Could you check a few things on this model? Use its own coordinates, in mm. A direction names the side the tool comes from. Round coordinates to 2 decimals unless told otherwise and drop trailing zeros. Loops run counter-clockwise (first coordinate to the right, second up) from the corner with the lowest first, then second, coordinate; pieces in that order, holes last. Notation, with made-up numbers: (39.25, 52.25) -> (67.25, 52.25) arc R28 cw to (67.25, 90.25) -> close; hole circle Ø10 at (-3.5, 8.5). An arc over 180 degrees is marked (long way). Put each result on its own line as item: value. Start each with the question number.
1. If we mould it in two halves opening along Y, with no side actions, what happens to faces 1 (the cylindrical face through (13.113, 25.145, 3.131)), 2 (the cylindrical face through (-30.235, -23.183, 3.131)), 3 (the flat face through (16, 1, 0))? For each: pulls with the +Y half, pulls with the -Y half, needs draft (parallel to the pull), parting line crosses it, or undercut.
2. I'm going to push flat-ended pins straight in: P1, Ø6, axis at x = 17, z = 13, coming from the +Y side; P2, Ø8.5, axis at x = -12.7, y = -22, coming from the +Z side; P3, Ø2, axis at x = -3, z = 11, coming from the +Y side. Where does each tip first touch, or does it pass through?
3. Imagine slicing it at D-D, the plane x = -25.4. Please give me the cut outline in (y, z) (3 decimals).
4. Which directions (+Z, -Z, +X, -X, +Y, -Y) give clear straight access to the entire face, cutting with the end or side of a thin tool? Please do faces 4 (the flat face through (16, -16, 6.35)), 5 (the cylindrical face through (-12.287, 25.145, 3.131)).
5. Imagine slicing it at A-A, the plane y = 0. Count the separate pieces of the cut face and the enclosed holes in it, and give its area (3 significant figures).
6. Imagine slicing it at B-B, the plane x = 0. Please give me the cut outline in (y, z), and give its area (3 significant figures).
7. I need wall thicknesses on line 1 (Y direction, x = 12.7, z = 5); line 2 (Y direction, x = 0, z = 12.5); line 3 (Z direction, x = 31, y = -19). Which ranges of each line are inside material? Lowest first, please. Write a range as [from, to].
```python
from build123d import *

# Parameters (mm, degrees)
SKETCH1_R           = 38.1
BOSS_EXTRUDE1_DEPTH = 6.35
SKETCH2_R           = 17.4625
BOSS_EXTRUDE2_DEPTH = 12.7
FILLET2_R           = 2.54
CUT_EXTRUDE1_REACH  = 59.15
SKETCH3_R           = 14.2875
SKETCH4_R           = 3.175
CUT_EXTRUDE2_DEPTH  = 58.15


with BuildPart() as part:
    # Sketch1 → Boss-Extrude1 (new body)
    with BuildSketch(Plane.XY):
        Circle(SKETCH1_R)
    extrude(amount=BOSS_EXTRUDE1_DEPTH)

    # Sketch2 → Boss-Extrude2 (add)
    with BuildSketch(Plane.XY.offset(6.35)):
        Circle(SKETCH2_R)
    extrude(amount=BOSS_EXTRUDE2_DEPTH)

    # Fillet2
    fillet2_edges = [part.edges().sort_by_distance(p)[0] for p in [
        (-17.4625, 0, 6.35),
    ]]
    fillet(fillet2_edges, radius=FILLET2_R)

    # Sketch3 → Cut-Extrude1 (cut, up to next)
    with BuildSketch(Plane.XY.offset(19.05), mode=Mode.PRIVATE) as cut_extrude1_sk1:
        Circle(SKETCH3_R)
    cut_extrude1_tool1 = extrude(cut_extrude1_sk1.sketch, amount=-CUT_EXTRUDE1_REACH, mode=Mode.PRIVATE) & part.part
    add(cut_extrude1_tool1.solids().sort_by_distance((0, 0, 19.05))[0], mode=Mode.SUBTRACT)

    # Sketch4 → Cut-Extrude2 (cut, through all)
    with BuildSketch(Plane(origin=(0, 0, 0), x_dir=(-1, 0, 0), z_dir=(0, 0, -1))):
        with Locations((-25.4, 0)):
            Circle(SKETCH4_R)
        with Locations((-12.7, 21.997045256)):
            Circle(SKETCH4_R)
        with Locations((12.7, 21.997045256)):
            Circle(SKETCH4_R)
        with Locations((25.4, 0)):
            Circle(SKETCH4_R)
        with Locations((12.7, -21.997045256)):
            Circle(SKETCH4_R)
        with Locations((-12.7, -21.997045256)):
            Circle(SKETCH4_R)
    extrude(amount=-CUT_EXTRUDE2_DEPTH, mode=Mode.SUBTRACT)


solid = part.part
```
Entries:
1. face 1: undercut
1. face 2: parting line crosses it
1. face 3: needs draft
2. P1: y = 10.44
2. P2: z = 6.35
2. P3: y = 17.35
3. outline: (-28.398, 0) -> (-3.175, 0) -> (-3.175, 6.35) -> (-28.398, 6.35) -> close; (3.175, 0) -> (28.398, 0) -> (28.398, 6.35) -> (3.175, 6.35) -> close
4. face 4: +Z
4. face 5: +Z, -Z
5. separate pieces: 4
5. enclosed holes: 0
5. area: 305 mm^2
6. outline: (-38.1, 0) -> (-14.29, 0) -> (-14.29, 19.05) -> (-17.46, 19.05) -> (-17.46, 8.89) arc R2.54 cw to (-20, 6.35) -> (-38.1, 6.35) -> close; (14.29, 0) -> (38.1, 0) -> (38.1, 6.35) -> (20, 6.35) arc R2.54 cw to (17.46, 8.89) -> (17.46, 19.05) -> (14.29, 19.05) -> close
6. area: 386 mm^2
7. line 1: [-35.92, -25.17], [-18.82, -6.55], [6.55, 18.82], [25.17, 35.92]
7. line 2: [-17.46, -14.29], [14.29, 17.46]
7. line 3: [0, 6.35]
